Verification items for the finished model (mm, model axes). Face numbers are marked on the shaded views. A direction names the side the tool comes from. Give positions to 0.01 mm unless a question says otherwise; leave off trailing zeros. Order: outer loops, then holes, each group sorted by start corner. A loop starts at its lowest first (then second) coordinate and runs counter-clockwise, first axis right, second up.
(1) Sectioned sample at B-B on y = 0. Record the cut outline in (x, z) (3 decimals), plus the area to 3 significant figures.
(2) Sectioned sample at A-A on x = 6.5. Record the cut outline in (y, z) (3 decimals).
(3) Access from +Z, -Z, +X, -X, +Y, -Y to the whole of each face (thin tool, end or side, straight path). Record for the marked faces 1 and 2.
(4) Sectioned sample at C-C on z = 4.25. Record the cut outline in (x, y) (3 decimals), plus the area to 3 significant figures.
(5) Mould release check, pull along Y, two halves, no side actions. Record for the marked faces 3, 4 and 5: pulls with the +Y half, pulls with the -Y half, needs draft (parallel to the pull), parting line crosses it, or undercut.
(6) Scan lines: L1, parallel to Y at x = 6.5, z = 4.5 (3 decimals); L2, parallel to Y at x = 6.5, z = -2 (3 decimals); L3, parallel to Z at x = 11, y = -8.25. Record each from-to range of solid material in increasing order.
(7) Gauge pin test, flat ends, axial feed: pin 1 (1 mm diameter, centred on x = 0.5, z = 7.5, fed in from -Y); pin 2 (4 mm diameter, centred on x = 3, z = -8.5, fed in from -Y); pin 3 (1.5 mm diameter, centred on x = -1, z = -5.5, fed in from +Y); pin 4 (5 mm diameter, centred on x = 6.5, y = 0, fed in from +Z). Record the tip position at first contact, or that the pin passes through.
Autodesk Inventor part; units mm, degrees
ref_plane "YZ Plane" through (0, 0, 0) normal (1, 0, 0) x (0, 1, 0)
ref_plane "XZ Plane" through (0, 0, 0) normal (0, 1, 0) x (-1, 0, 0)
ref_plane "XY Plane" through (0, 0, 0) normal (0, 0, 1) x (1, 0, 0)
sketch "Sketch1" plane through (0, 0, 0) normal (0, 1, 0) x (-1, 0, 0)
  line L0 (0, 0) -> (0, -2.5)
  line L1 (3.5, 0.5) -> (0, 0)
  line L2 (3.5, -3) -> (0, -2.5)
  line L3 (3.5, -3) -> (3.5, -14.25)
  line L4 (3.5, -14.25) -> (-6.5, -14.25)
  line L5 (3.5, 0.5) -> (3.5, 11.75)
  line L6 (3.5, 11.75) -> (-6.5, 11.75)
  line L7 (-6.5, 11.75) -> (-6.5, -14.25)
  dimension "d0" = 2.5
  dimension "d6" = 3.5
  dimension "d9" = 11.25
  dimension "d11" = 10
  dimension "d12" = 90
  dimension "d13" = 11.25
  dimension "d15" = 10
  dimension "d16" = 90
  dimension "d17" = 3.5
  dimension "d18" = 11.75
revolve "Revolution1" add sketch "Sketch1" angle 360 about axis through (6.5, 0, 11.75) along (0, 0, -1)
sketch "Sketch2" plane through (6.5, 0, -14.25) normal (0, 0, -1) x (-1, 0, 0)
  circle A0 centre (0, 0) radius 2.975
  circle A1 centre (0, 0) radius 10
  point P0 (6.5, 0)
  dimension "d20" = 5.95
extrude "Extrusion1" cut sketch "Sketch2" against normal blind 26 contours A0
properties part number "roller" material "ABS Plastic"
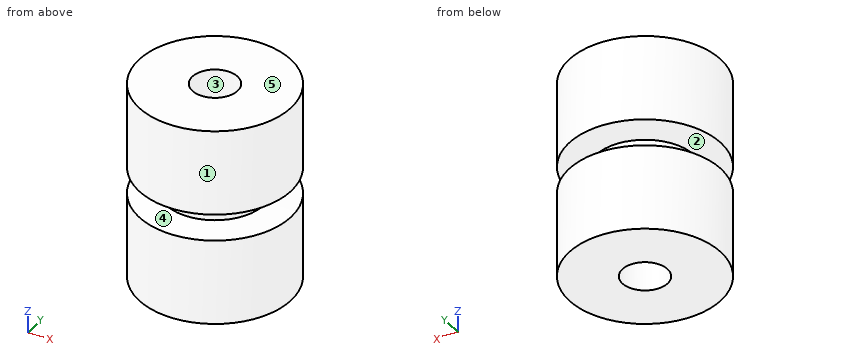
Ans:
1. outline: (-3.5, -14.25) - (3.525, -14.25) - (3.525, 11.75) - (-3.5, 11.75) - (-3.5, 0.5) - (0, 0) - (0, -2.5) - (-3.5, -3) - close; (9.475, -14.25) - (16.5, -14.25) - (16.5, -3) - (13, -2.5) - (13, 0) - (16.5, 0.5) - (16.5, 11.75) - (9.475, 11.75) - close
1. area: 344 mm2
2. outline: (-10, -14.25) - (-2.975, -14.25) - (-2.975, 11.75) - (-10, 11.75) - (-10, 0.5) - (-6.5, 0) - (-6.5, -2.5) - (-10, -3) - close; (2.975, -14.25) - (10, -14.25) - (10, -3) - (6.5, -2.5) - (6.5, 0) - (10, 0.5) - (10, 11.75) - (2.975, 11.75) - close
3. face 1: +Z, -Z
3. face 2: none
4. outline: circle Ø20 at (6.5, 0); hole circle Ø5.95 at (6.5, 0)
4. area: 286 mm2
5. face 3: undercut
5. face 4: parting line crosses it
5. face 5: needs draft
6. L1: y = -10 to -2.975, 2.975 to 10
6. L2: y = -6.5 to -2.975, 2.975 to 6.5
6. L3: z = -14.25 to -2.91, 0.41 to 11.75
7. pin 1: stops at y = -8.35
7. pin 2: stops at y = -9.89
7. pin 3: stops at y = 7.38
7. pin 4: passes through
